from build123d import *

# Parameters (mm, degrees)
SKETCH1_W           = 76.2
SKETCH1_H           = 50.8
BOSS_EXTRUDE1_DEPTH = 31.75
SKETCH4_W           = 12.7
SKETCH4_H           = 12.7


with BuildPart() as part:
    # Sketch1 → Boss-Extrude1 (new body, symmetric)
    with BuildSketch(Plane.XY):
        with Locations((38.1, 25.4)):
            Rectangle(SKETCH1_W, SKETCH1_H)
    extrude(amount=BOSS_EXTRUDE1_DEPTH, both=True)

    # Sketch3 → Revolve1 (revolve)
    with BuildSketch(Plane.XY):
        with BuildLine():
            Line((12.7, 0), (12.7, -12.7))
            Line((12.7, -12.7), (8.89, -12.7))
            Line((8.89, -12.7), (8.89, -28.575))
            ThreePointArc((8.89, -28.575), (13.599228719, -31.3489681), (19.05, -31.75))
            Line((19.05, -31.75), (19.05, -28.575))
            Line((19.05, -28.575), (19.05, 0))
            Line((19.05, 0), (12.7, 0))
        make_face()
    revolve(axis=Axis((19.05, -28.575, 0), (0, 1, 0)))

    # Sketch4 → Revolve2 (revolve)
    with BuildSketch(Plane.XY):
        with Locations((50.8, -6.35)):
            Rectangle(SKETCH4_W, SKETCH4_H)
    revolve(axis=Axis((57.15, 0, 0), (0, -1, 0)))


solid = part.part
Part model, mm, in its own coordinate system. A direction names the side the tool comes from. Give positions to 0.01 mm unless a question says otherwise; leave off trailing zeros. Loops run counter-clockwise (first coordinate to the right, second up) from the corner with the lowest first, then second, coordinate; pieces in that order, holes last. Notation, with made-up numbers: M 50,-1.75 L 75,-1.75 A22 ccw 75,13.25 Z; hole C 35,60 d11. An arc over 180 degrees is marked long. Put each result on its own line as item: value. Start each with the question number.
1) Saw through at D-D (x = 30.5). List the corners of the cut face in (y, z).
2) Saw through at A-A (x = 57.15). List the corners of the cut face in (y, z), then the cut area to 3 significant figures.
3) Saw through at C-C (z = 22). List the corners of the cut face in (x, y).
4) 3-axis set-ups, long thin cutter, end or side, ignore diameter. For faces 1 (the flat face through (26, -12.7, 0)), 2 (the flat face through (38, 26, 31.75)), 3 (the flat face through (57, -12.7, 0)), 4 (the cylindrical face through (9.36, -20.75, 3.05)): which of +Z, -Z, +X, -X, +Y, -Y reach the whole face in a straight line?
5) Saw through at B-B (y = -20). List the corners of the cut face in (x, z).
6) Flat gauge pins, fed straight in: pin 1 (1.5 mm diameter, centred on x = 29.5, z = 7.5, fed in from -Y); pin 2 (1 mm diameter, centred on x = 62, y = -5, fed in from +Z); pin 3 (8 mm diameter, centred on x = 48.5, z = 5.5, fed in from -Y). Where does each tip first touch, or does it go through?
7) Pull direction X, two halves, no side cores. Call faces 5 (the cylindrical face through (25.394, -6.439, 0.279)), 6 (the flat face through (76.2, 25, 0)), 7 (the flat face through (38, 26, -31.75)): +X half, -X half, draft (parallel to the pull), parting line (faces both ways), or undercut.
8) Probe probe 1 along Y at (x, z) = (66, 27.5); probe 2 along Y at (x, z) = (64.5, 8); probe 3 along X at (y, z) = (-3, 4). List the from-to ranges inside material, lowest first.
Numbers:
1. outline: M 0,-31.75 L 50.8,-31.75 L 50.8,31.75 L 0,31.75 Z
2. outline: M -12.7,-12.7 L 0,-12.7 L 0,-31.75 L 50.8,-31.75 L 50.8,31.75 L 0,31.75 L 0,12.7 L -12.7,12.7 Z
2. area: 3,550 mm^2
3. outline: M 0,0 L 76.2,0 L 76.2,50.8 L 0,50.8 Z
4. face 1: none
4. face 2: +Z, +X, -X, +Y, -Y
4. face 3: +Z, -Z, +X, -Y
4. face 4: -Y
5. outline: C 19.05,0 d20.32
6. pin 1: y = 0
6. pin 2: z = 11.93
6. pin 3: y = -12.7
7. face 5: undercut
7. face 6: +X half
7. face 7: draft
8. probe 1: 0 to 50.8
8. probe 2: -12.7 to 50.8
8. probe 3: 14.12 to 23.98, 45.1 to 69.2
